Geometry check sheet. Reference: the model listing, model coordinates, mm. Face numbers are marked on the shaded views. Coordinates: 2 decimals unless noted, no trailing zeros. Order: outer loops, then holes, each group sorted by start corner. A loop starts at its lowest first (then second) coordinate and runs counter-clockwise, first axis right, second up. Notation, with made-up numbers: (83, 58.25) - (97, 58.25) arc R19 cw to (97, 82.25) - close; hole circle Ø3 at (-37.75, 2). An arc over 180 degrees is marked (long way). Use CSV: the item, a comma, the result in double quotes. Start each with the question number.
1) Sectioned sample at C-C, the plane x = -17.5. Record the cut outline in (y, z), and give its area (3 significant figures).
2) Sectioned sample at B-B, the plane y = 1.05. Count the separate pieces of the cut face and the enclosed holes in it, and give its area (3 significant figures).
3) Draft check along X on the marked faces 1, 2, 3 and 4. Enter one of: released by +X, released by -X, zero draft, split by the parting line, or undercut.
4) Thickness scan on probe 1 along Z at (x, y) = (-17.5, 3.35); probe 2 along Z at (x, y) = (29, 2.95); probe 3 along X at (y, z) = (2.35, -10.4). Record the ranges inside material, lowest first. Write a range as [from, to].
5) Depth check by flat-ended pin: P1, Ø1.2, axis at x = -34, z = -10.4, coming from the -Y side; P2, Ø3, axis at x = 29, z = -13.4, coming from the +Y side. Enter the tip coordinate at first touch or a pass-through.
6) Sectioned sample at A-A, the plane x = 15.6. Record the cut outline in (y, z).
7) Sectioned sample at D-D, the plane z = -3. Record the cut outline in (x, y).
from build123d import *

# Parameters (mm, degrees)
SKETCH1_W           = 98
SKETCH1_H           = 30
SKETCH1_R           = 7
SKETCH1_R_2         = 1
BOSS_EXTRUDE1_DEPTH = 5.9
SKETCH4_R           = 7
SKETCH4_R_2         = 1
CUT_EXTRUDE3_DEPTH  = 10
FILLET1_R           = 10
SKETCH5_R           = 2.05
CUT_EXTRUDE4_DEPTH  = 10


with BuildPart() as part:
    # Sketch1 → Boss-Extrude1 (new body)
    with BuildSketch(Plane(origin=(0, 0, 0), x_dir=(1, 0, 0), z_dir=(0, 1, 0))):
        Rectangle(SKETCH1_W, SKETCH1_H)
        with Locations((-34, 0)):
            Circle(SKETCH1_R, mode=Mode.SUBTRACT)
        with Locations((-44.4, 0)):
            Circle(SKETCH1_R_2, mode=Mode.SUBTRACT)
        with Locations((-47.4, 0)):
            Circle(SKETCH1_R_2, mode=Mode.SUBTRACT)
        with Locations((-34, 10.4)):
            Circle(SKETCH1_R_2, mode=Mode.SUBTRACT)
        with Locations((-34, 13.4)):
            Circle(SKETCH1_R_2, mode=Mode.SUBTRACT)
        with Locations((-23.6, 0)):
            Circle(SKETCH1_R_2, mode=Mode.SUBTRACT)
        with Locations((-20.6, 0)):
            Circle(SKETCH1_R_2, mode=Mode.SUBTRACT)
        with Locations((-34, -10.4)):
            Circle(SKETCH1_R_2, mode=Mode.SUBTRACT)
        with Locations((-34, -13.4)):
            Circle(SKETCH1_R_2, mode=Mode.SUBTRACT)
    extrude(amount=BOSS_EXTRUDE1_DEPTH)

    # Sketch4 → Cut-Extrude3 (cut)
    with BuildSketch(Plane(origin=(0, 5.9, 0), x_dir=(1, 0, 0), z_dir=(0, 1, 0))):
        with Locations((-34, 0)):
            Circle(SKETCH4_R)
        with Locations((-34, -13.4)):
            Circle(SKETCH4_R_2)
        with Locations((-34, -10.4)):
            Circle(SKETCH4_R_2)
        with Locations((-44.4, 0)):
            Circle(SKETCH4_R_2)
        with Locations((-47.4, 0)):
            Circle(SKETCH4_R_2)
        with Locations((-34, 13.4)):
            Circle(SKETCH4_R_2)
        with Locations((-23.6, 0)):
            Circle(SKETCH4_R_2)
        with Locations((-20.6, 0)):
            Circle(SKETCH4_R_2)
        with Locations((-34, 10.4)):
            Circle(SKETCH4_R_2)
        with Locations((29, -13.4)):
            Circle(SKETCH4_R_2)
        with Locations((29, -10.4)):
            Circle(SKETCH4_R_2)
        with Locations((42.4, 0)):
            Circle(SKETCH4_R_2)
        with Locations((39.4, 0)):
            Circle(SKETCH4_R_2)
        with Locations((29, 0)):
            Circle(SKETCH4_R)
        with Locations((29, 10.4)):
            Circle(SKETCH4_R_2)
        with Locations((29, 13.4)):
            Circle(SKETCH4_R_2)
        with Locations((18.6, 0)):
            Circle(SKETCH4_R_2)
        with Locations((15.6, 0)):
            Circle(SKETCH4_R_2)
    extrude(amount=-CUT_EXTRUDE3_DEPTH, mode=Mode.SUBTRACT)

    # Fillet1
    fillet1_edges = [part.edges().sort_by_distance(p)[0] for p in [
        (49, 2.95, 15),
        (-49, 2.95, 15),
        (-49, 2.95, -15),
        (49, 2.95, -15),
    ]]
    fillet(fillet1_edges, radius=FILLET1_R)

    # Sketch5 → Cut-Extrude4 (cut)
    with BuildSketch(Plane(origin=(0, 5.9, 0), x_dir=(1, 0, 0), z_dir=(0, 1, 0))):
        with Locations((-17.5, 10)):
            Circle(SKETCH5_R)
        with Locations((-17.5, -10)):
            Circle(SKETCH5_R)
        with Locations((4.5, -10)):
            Circle(SKETCH5_R)
        with Locations((4.5, 10)):
            Circle(SKETCH5_R)
    extrude(amount=-CUT_EXTRUDE4_DEPTH, mode=Mode.SUBTRACT)


solid = part.part
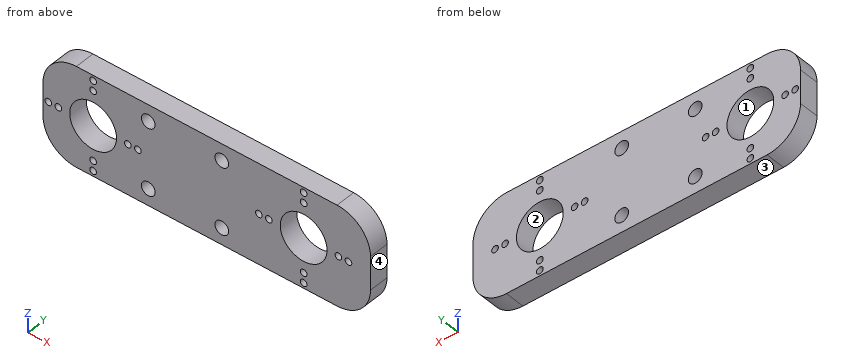
Evaluation:
1,outline,"(0, -15) - (5.9, -15) - (5.9, -12.05) - (0, -12.05) - close; (0, -7.95) - (5.9, -7.95) - (5.9, 7.95) - (0, 7.95) - close; (0, 12.05) - (5.9, 12.05) - (5.9, 15) - (0, 15) - close"
1,area,"129 mm²"
2,separate pieces,"1"
2,enclosed holes,"22"
2,area,"2,440 mm²"
3,face 1,"undercut"
3,face 2,"undercut"
3,face 3,"zero draft"
3,face 4,"released by +X"
4,probe 1,"[-15, -12.05], [-7.95, 7.95], [12.05, 15]"
4,probe 2,"[-15, -14.4], [-12.4, -11.4], [-9.4, -7], [7, 9.4], [11.4, 12.4], [14.4, 15]"
4,probe 3,"[-47.42, -35], [-33, -19.51], [-15.49, 2.49], [6.51, 28], [30, 47.42]"
5,P1,"through"
5,P2,"y = 5.9"
6,outline,"(0, -15) - (5.9, -15) - (5.9, -1) - (0, -1) - close; (0, 1) - (5.9, 1) - (5.9, 15) - (0, 15) - close"
7,outline,"(-49, 0) - (-40.32, 0) - (-40.32, 5.9) - (-49, 5.9) - close; (-27.68, 0) - (22.68, 0) - (22.68, 5.9) - (-27.68, 5.9) - close; (35.32, 0) - (49, 0) - (49, 5.9) - (35.32, 5.9) - close"
